The listing builds one solid part. Answer for the finished solid, in the listing's coordinates (mm). Face numbers are marked on the shaded views. Coordinates: 2 decimals unless noted, no trailing zeros. Order: outer loops, then holes, each group sorted by start corner. A loop starts at its lowest first (then second) coordinate and runs counter-clockwise, first axis right, second up. Notation, with made-up numbers: (2, 53) -> (39, 53) arc R18 cw to (39, 84) -> close; hole circle Ø1 at (66, 82.5). An arc over 180 degrees is marked (long way). Return JSON: item names as keys, results as strings.
```python
from build123d import *

# Parameters (mm, degrees)
SKETCH1_W                    = 70
SKETCH1_H                    = 25
BASE_FLANGE1_DEPTH           = 1.5
EDGE_FLANGE1_DEPTH           = 10
EDGE_FLANGE2_STRIP_CUT_DEPTH = 25
EDGE_FLANGE2_DEPTH           = 25
EDGE_FLANGE3_STRIP_CUT_DEPTH = 25
EDGE_FLANGE3_DEPTH           = 25


# Sheet-metal steps are written as plain solids
with BuildPart() as part:
    # Sketch1 → Base-Flange1 (new body)
    with BuildSketch(Plane(origin=(0, 0, 0), x_dir=(1, 0, 0), z_dir=(0, 1, 0))):
        Rectangle(SKETCH1_W, SKETCH1_H)
    extrude(amount=-BASE_FLANGE1_DEPTH)

    # Edge-Flange1 section (across the edge) → Edge-Flange1 (add)
    with BuildSketch(Plane(origin=(-35.129882454, 0, -5), x_dir=(0.3420201433256639, 0.9396926207859102, 0), z_dir=(0, 0, 1))):
        with BuildLine():
            Line((-1.5, 0.129882454), (-1.5, 24.735509529))
            Line((-1.5, 24.735509529), (0, 24.735509529))
            Line((0, 24.735509529), (0, 0.129882454))
            ThreePointArc((0, 0.129882454), (0.011190609, 0.001973206), (0.044422416, -0.122049584))
            Line((0.044422416, -0.122049584), (-1.365116516, -0.635079799))
            ThreePointArc((-1.365116516, -0.635079799), (-1.46602102, -0.25849906), (-1.5, 0.129882454))
        make_face()
    extrude(amount=EDGE_FLANGE1_DEPTH)

    # Edge-Flange2 strip (across the edge) → Edge-Flange2 strip cut (cut)
    with BuildSketch(Plane(origin=(35, 0, 12.5), x_dir=(-0.49999999999999495, 0.8660254037844416, 0), z_dir=(0, 0, -1))):
        Polygon((-4.936952418, 5.551052423), (-1.200352418, -0.920928625), (0.098685688, -0.170928625), (-3.637914312, 6.301052423), align=None)
    extrude(amount=EDGE_FLANGE2_STRIP_CUT_DEPTH, mode=Mode.SUBTRACT)

    # Edge-Flange2 section (across the edge) → Edge-Flange2 (add)
    with BuildSketch(Plane(origin=(35, 0, 12.5), x_dir=(-0.49999999999999495, 0.8660254037844416, 0), z_dir=(0, 0, -1))):
        with BuildLine():
            Line((-1.5, 0.197371375), (-1.5, 79.598076211))
            Line((-1.5, 79.598076211), (0, 79.598076211))
            Line((0, 79.598076211), (0, 0.197371375))
            ThreePointArc((0, 0.197371375), (0.025099036, 0.006725267), (0.098685688, -0.170928625))
            Line((0.098685688, -0.170928625), (-1.200352418, -0.920928625))
            ThreePointArc((-1.200352418, -0.920928625), (-1.423789703, -0.381503301), (-1.5, 0.197371375))
        make_face()
    extrude(amount=EDGE_FLANGE2_DEPTH)

    # Edge-Flange3 strip (across the edge) → Edge-Flange3 strip cut (cut)
    with BuildSketch(Plane(origin=(103.933956091, 39.799038106, 12.5), x_dir=(-0.8191520442889849, 0.573576436351056, 0), z_dir=(0, 0, -1))):
        Polygon((-4.44875879, 5.991091638), (-1.290447996, -0.781927716), (0.069013684, -0.148000323), (-3.08929711, 6.625019031), align=None)
    extrude(amount=EDGE_FLANGE3_STRIP_CUT_DEPTH, mode=Mode.SUBTRACT)

    # Edge-Flange3 section (across the edge) → Edge-Flange3 (add)
    with BuildSketch(Plane(origin=(103.933956091, 39.799038106, 12.5), x_dir=(-0.8191520442889849, 0.573576436351056, 0), z_dir=(0, 0, -1))):
        with BuildLine():
            Line((-1.5, 0.163300289), (-1.5, 44.667458006))
            Line((-1.5, 44.667458006), (0, 44.667458006))
            Line((0, 44.667458006), (0, 0.163300289))
            ThreePointArc((0, 0.163300289), (0.017460361, 0.003870869), (0.069013684, -0.148000323))
            Line((0.069013684, -0.148000323), (-1.290447996, -0.781927716))
            ThreePointArc((-1.290447996, -0.781927716), (-1.44698365, -0.320788552), (-1.5, 0.163300289))
        make_face()
    extrude(amount=EDGE_FLANGE3_DEPTH)


solid = part.part
```
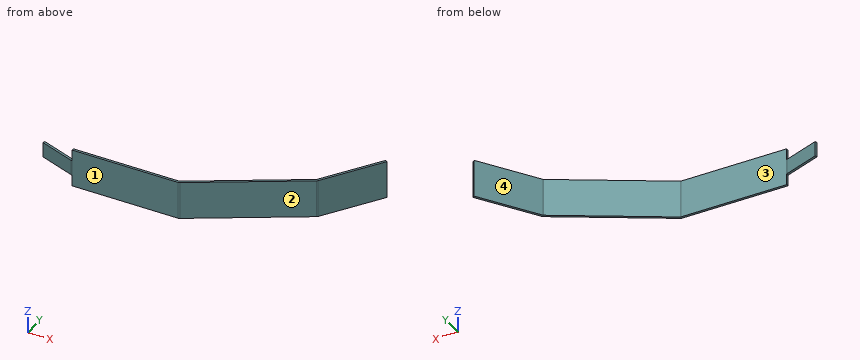
Item 1: Flat-ended cylindrical pins translate along their axes: pin 1 (3 mm diameter, centred on y = 64.5, z = -3, fed in from -X); pin 2 (5 mm diameter, centred on x = -52, y = 3.5, fed in from +Z); pin 3 (12.5 mm diameter, centred on x = -15.5, z = -1, fed in from +Y). Find the tip coordinate at first contact, or state that the pin passes through.
Answer list:
{"pin 1": "x = 120.18", "pin 2": "z = 5", "pin 3": "y = 0"}
Item 2: Determine the mould class of the marked faces 1, 2, 3 and 4 for opening direction X: pulls with the +X half, pulls with the -X half, needs draft (parallel to the pull), parting line crosses it, or undercut.
Answer list:
{"face 1": "needs draft", "face 2": "pulls with the +X half", "face 3": "undercut", "face 4": "pulls with the -X half"}
Item 3: The part is cut by section A-A on z = 0. Determine the outline of the cut face in (x, y), plus the area to 3 significant figures.
Answer list:
{"outline": "(-58.89, 7.05) -> (-35.76, -1.37) arc R2.24 ccw to (-35, -1.5) -> (34.8, -1.5) arc R2.24 ccw to (35.92, -1.2) -> (104.54, 38.42) arc R2.24 ccw to (105.26, 39.07) -> (130.78, 75.53) -> (129.55, 76.39) -> (104.03, 39.93) arc R0.74 cw to (103.79, 39.72) -> (35.17, 0.1) arc R0.74 cw to (34.8, 0) -> (-35, 0) arc R0.74 cw to (-35.25, 0.04) -> (-58.37, 8.46) -> close", "area": "330 mm2"}
Item 4: The part is cut by section B-B on x = -16. Determine the outline of the cut face in (y, z).
Answer list:
{"outline": "(-1.5, -12.5) -> (0, -12.5) -> (0, 12.5) -> (-1.5, 12.5) -> close"}
Item 5: Find the intervals of material crossed by probe 1 along Y at (x, z) = (-2.5, -7.25); probe 2 along X at (y, z) = (49, -8.5); probe 3 along Y at (x, z) = (61, 11.25), in increasing order.
Answer list:
{"probe 1": "-1.5 to 0", "probe 2": "110.38 to 112.21", "probe 3": "13.28 to 15.01"}
Item 6: The part is cut by section C-C on y = 24. Determine the outline of the cut face in (x, z).
Answer list:
{"outline": "(76.57, -12.5) -> (79.57, -12.5) -> (79.57, 12.5) -> (76.57, 12.5) -> close"}
